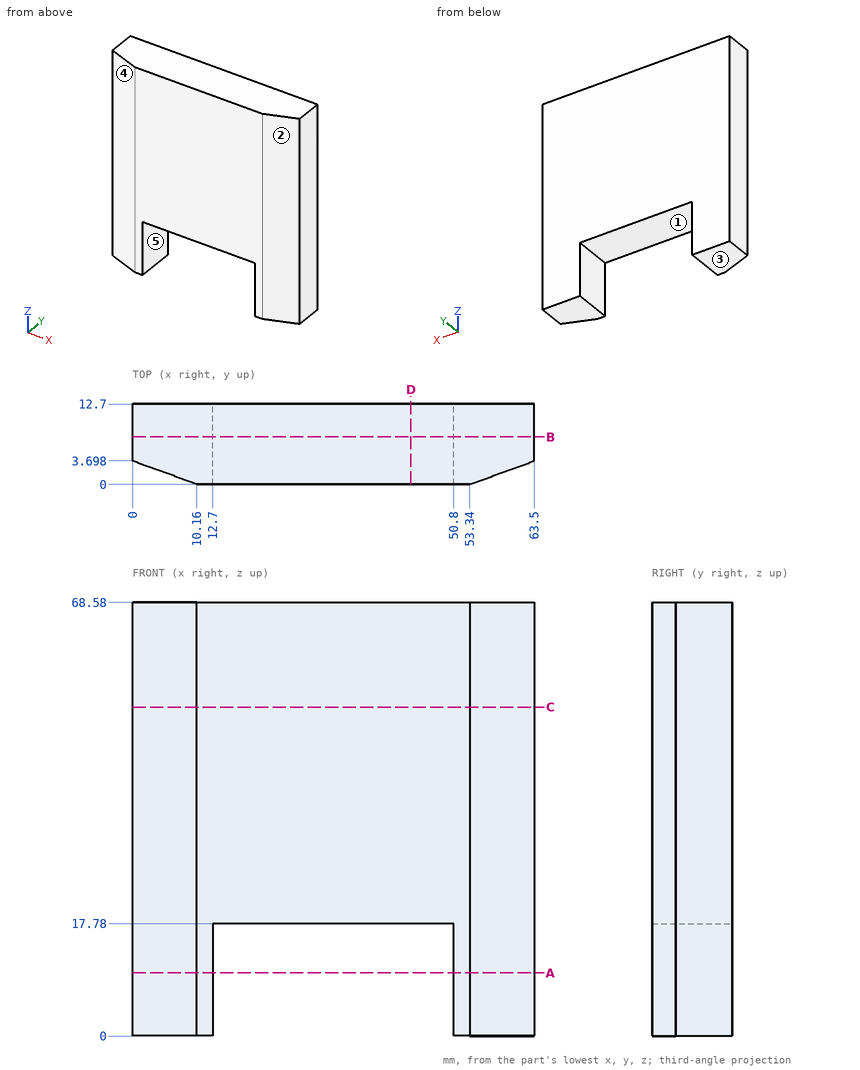
For this review, use the dimensioned drawing (mm, ordinates from the lowest corner) and the shaded views. A direction names the side the tool comes from. Give positions to 0.01 mm unless a question says otherwise; leave off trailing zeros. Write each loop counter-clockwise with the first axis right and the second up, starting at its lowest first coordinate (ties: lowest second). Pieces come first, ordered by that corner, then holes. Notation, with made-up numbers: M 23.25,82 L 30.25,82 A35 ccw 30.25,117 Z; hole C 55.25,-2 d10. An arc over 180 degrees is marked long. Answer as a JSON object with one key per item and string values. Group by question number.
1) Clearance check with a flat-ended pin moving along its axis: pin 1 Ø5 at (x, y) = (38, 5.5) entering from -Z. State where the tip first meets the part, or that it passes through.
2) For line 1 along X through (y, z) = (7.25, 16); line 2 along Z through (x, y) = (26.5, 7.75); line 3 along Y through (x, z) = (9, 55.5), list the stretches that pass through material, from the lowest coordinate up.
3) Mouldability with a two-part tool opening along X and no side actions: class the marked faces 1, 2 and 3 as released by +X, released by -X, zero draft, split by the parting line, or undercut.
4) We need section A-A (z = 10). Give the boundary of the cut face in (x, y).
5) We need section D-D (x = 44). Give the boundary of the cut face in (y, z).
6) We need section B-B (y = 7.5). Give the boundary of the cut face in (x, z).
7) Tool access review of the marked faces 4 and 5: name each direction out of +Z, -Z, +X, -X, +Y, -Y from which nothing blocks a thin tool from reaching the whole face with its end or side.
8) We need section C-C (z = 52). Give the boundary of the cut face in (x, y), and give its area (3 significant figures).
Answer key:
{
 "1": {"pin 1": "stops at z = 17.78"},
 "2": {"line 1": "x = 0 to 12.7, 50.8 to 63.5", "line 2": "z = 17.78 to 68.58", "line 3": "y = 0.42 to 12.7"},
 "3": {"face 1": "undercut", "face 2": "released by +X", "face 3": "zero draft"},
 "4": {"outline": "M 0,3.7 L 10.16,0 L 12.7,0 L 12.7,12.7 L 0,12.7 Z; M 50.8,0 L 53.34,0 L 63.5,3.7 L 63.5,12.7 L 50.8,12.7 Z"},
 "5": {"outline": "M 0,17.78 L 12.7,17.78 L 12.7,68.58 L 0,68.58 Z"},
 "6": {"outline": "M 0,0 L 12.7,0 L 12.7,17.78 L 50.8,17.78 L 50.8,0 L 63.5,0 L 63.5,68.58 L 0,68.58 Z"},
 "7": {"face 4": "+Z, -Z, -X, -Y", "face 5": "-Z, +Y, -Y"},
 "8": {"outline": "M 0,3.7 L 10.16,0 L 53.34,0 L 63.5,3.7 L 63.5,12.7 L 0,12.7 Z", "area": "769 mm²"}
}
